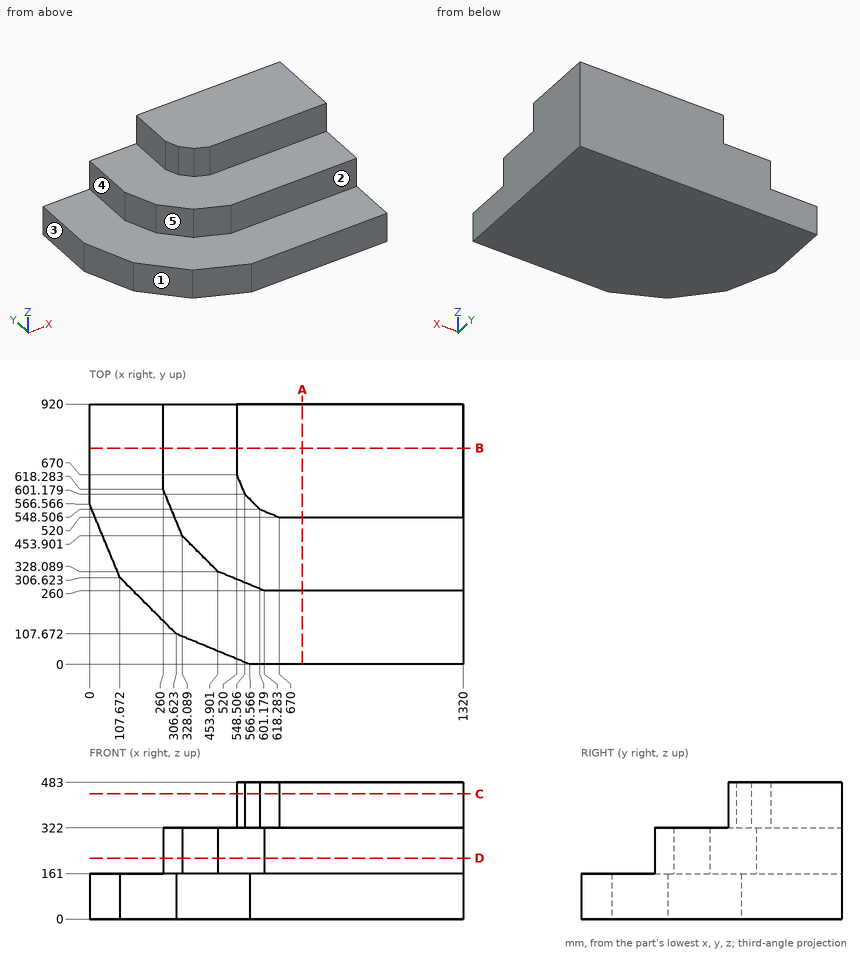
Design review of the part shown in the three views and the two pictorial views. Dimensions are in mm from the part's minimum x, y and z. A direction names the side the tool comes from. Give positions to 0.01 mm unless a question says otherwise; leave off trailing zeros. Order: outer loops, then holes, each group sorted by start corner. A loop starts at its lowest first (then second) coordinate and runs counter-clockwise, first axis right, second up. Notation, with made-up numbers: M -23.75,33 L -19.75,33 A20 cw -19.75,66 Z; hole C 17.25,23.25 d4. An arc over 180 degrees is marked long. Answer in a Markdown table with one row per item. Add a question column.
(1) Wall thickness on probe 1 along Z at (x, y) = (563, 282); probe 2 along Y at (x, z) = (682, 301); probe 3 along Z at (x, y) = (323.5, 796): over which ranges is each line inside the solid? List them lowest first. Write a range as [from, to].
(2) For pin 1 (4 mm diameter, centred on x = 514, y = 323, fed in from +Z); pin 2 (3 mm diameter, centred on y = 370.5, z = 219, fed in from -X); pin 3 (1 mm diameter, centred on x = 325, y = 404, fed in from +Z), all flat-tipped, find the tip position at first contact; note any pin that passes through.
(3) Consider section A-A on x = 752.5. State the section outline as (y, z) points.
(4) Consider section C-C on z = 442.5. State the section outline as (x, y) points.
(5) Consider section D-D on z = 215.5. State the section outline as (x, y) points.
(6) Consider section B-B on y = 764. State the section outline as (x, z) points, and give its area (3 significant figures).
(7) For the marked faces 1, 2, 3, 4 and 5, list the 3-axis set-ups (+Z, -Z, +X, -X, +Y, -Y) from which the entire face can be reached by the end or side of a thin tool; tool diameter is ignored.
Evaluation:
| question | item | result |
|---|---|---|
| 1 | probe 1 | z = [0, 161] |
| 1 | probe 2 | y = [260, 920] |
| 1 | probe 3 | z = [0, 322] |
| 2 | pin 1 | stops at z = 322 |
| 2 | pin 2 | stops at x = 409.99 |
| 2 | pin 3 | stops at z = 161 |
| 3 | outline | M 0,0 L 920,0 L 920,483 L 520,483 L 520,322 L 260,322 L 260,161 L 0,161 Z |
| 4 | outline | M 520,670 L 548.51,601.18 L 601.18,548.51 L 670,520 L 1320,520 L 1320,920 L 520,920 Z |
| 5 | outline | M 260,618.28 L 328.09,453.9 L 453.9,328.09 L 618.28,260 L 1320,260 L 1320,920 L 260,920 Z |
| 6 | outline | M 0,0 L 1320,0 L 1320,483 L 520,483 L 520,322 L 260,322 L 260,161 L 0,161 Z |
| 6 | area | 512,000 mm^2 |
| 7 | face 1 | +Z, -Z, -X, -Y |
| 7 | face 2 | +Z, +X, -X, -Y |
| 7 | face 3 | +Z, -Z, -X, +Y, -Y |
| 7 | face 4 | +Z, -X, +Y, -Y |
| 7 | face 5 | +Z, -X, -Y |
